The model under review builds one solid part; all positions refer to its coordinate system, in mm. Face numbers are marked on the shaded views. A direction names the side the tool comes from. Give positions to 0.01 mm unless a question says otherwise; leave off trailing zeros. Order: outer loops, then holes, each group sorted by start corner. A loop starts at its lowest first (then second) coordinate and runs counter-clockwise, first axis right, second up.
```python
from build123d import *

# Parameters (mm, degrees)
F1_DEPTH = 82.75
F2_SIZE  = 5
F3_R     = 31
F4_DEPTH = 33
F5_SIZE  = 2
F6_R     = 11.6
F7_DEPTH = 31.5
F8_R     = 32.5
F9_DEPTH = 28
F9_TAPER = 5
F11_D    = 6.6


with BuildPart() as f1:
    # F0 (on Top) → F1 (new body, symmetric)
    with BuildSketch(Plane.XY):
        Polygon((0, 37), (-55, 37), (-55, 25.5), (-40, 25.5), (-40, -36), (0, -36), (40, -36), (40, 25.5), (55, 25.5), (55, 37), align=None)
    extrude(amount=F1_DEPTH, both=True)

    # F2
    f2_edges = [f1.edges().sort_by_distance(p)[0] for p in [
        (40, -36, 0),
        (-40, -36, 0),
    ]]
    chamfer(f2_edges, length=F2_SIZE)

    # F3 (on face) → F4 (join)
    with BuildSketch(Plane(origin=(0, 0, -82.75), x_dir=(1, 0, 0), z_dir=(0, 0, -1))):
        Circle(F3_R)
    extrude(amount=F4_DEPTH)

    # F5
    f5_edges = [f1.edges().sort_by_distance(p)[0] for p in [
        (-31, 0, -115.75),
    ]]
    chamfer(f5_edges, length=F5_SIZE)

    # F6 (on face) → F7 (join)
    with BuildSketch(Plane(origin=(0, 0, -115.75), x_dir=(1, 0, 0), z_dir=(0, 0, -1))):
        Circle(F6_R)
    extrude(amount=F7_DEPTH)

    # F8 (on face) → F9 (join)
    with BuildSketch(Plane.XY.offset(82.75)):
        Circle(F8_R)
    extrude(amount=F9_DEPTH, taper=F9_TAPER)

    # F11 (through all)
    with Locations(Plane.XZ.offset(-25.5)):
        with Locations((-47.5, 52.25), (-47.5, 17.25), (-47.5, -17.75), (-47.5, -52.75), (47.5, 52.25), (47.5, 17.25), (47.5, -17.75), (47.5, -52.75)):
            Hole(F11_D / 2)


solid = f1.part
```
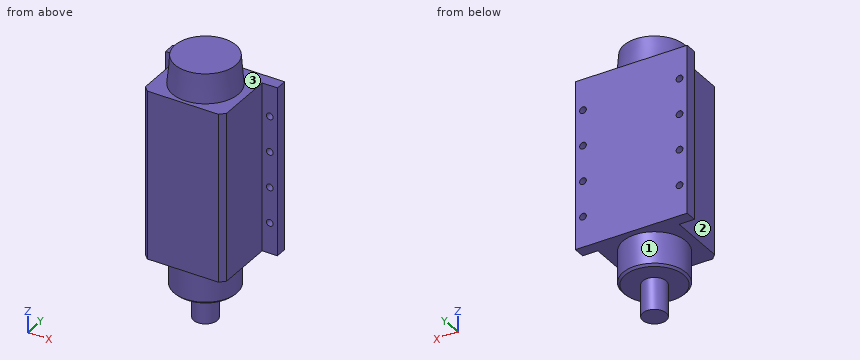
1. Take a section at D-D (z = -39). Write out the cut boundary in (x, y).
2. Take a section at A-A (z = 17.25). Write out the cut boundary in (x, y).
3. For the marked faces 1, 2 and 3, list the 3-axis set-ups (+Z, -Z, +X, -X, +Y, -Y) from which the entire face can be reached by the end or side of a thin tool; tool diameter is ignored.
4. Take a section at B-B (x = -47.5). Write out the cut boundary in (y, z), and give its area (3 significant figures).
5. To check wall thickness, follow line 1 (Z direction, x = -47, y = 30); line 2 (X direction, y = 34, z = 17); line 3 (X direction, y = 31, z = -17). State the ranges of each line that lie inside material, in increasing order.
6. Insertion check: pin 1 (8.5 mm diameter, centred on x = -47.5, z = 52.25, fed in from -Y); pin 2 (4 mm diameter, centred on x = 47.5, z = 52.25, fed in from -Y); pin 3 (5 mm diameter, centred on x = -36, y = -28, fed in from -Z); pin 4 (16.5 mm diameter, centred on x = -47.5, z = 24, fed in from -Y). Each pin has a flat end and moves straight along its axis. Give the tip position at first contact, or say it passes through.
7. Take a section at C-C (y = 0). Write out the cut boundary in (x, z), and give its area (3 significant figures).
Answer:
1. outline: (-55, 25.5) - (-40, 25.5) - (-40, -31) - (-35, -36) - (35, -36) - (40, -31) - (40, 25.5) - (55, 25.5) - (55, 37) - (-55, 37) - close
2. outline: (-55, 25.5) - (-50.8, 25.5) - (-50.8, 37) - (-55, 37) - close; (-44.2, 25.5) - (-40, 25.5) - (-40, -31) - (-35, -36) - (35, -36) - (40, -31) - (40, 25.5) - (44.2, 25.5) - (44.2, 37) - (-44.2, 37) - close; (50.8, 25.5) - (55, 25.5) - (55, 37) - (50.8, 37) - close
3. face 1: -Z
3. face 2: +Z, -Z, -X, -Y
3. face 3: +Z
4. outline: (25.5, -82.75) - (37, -82.75) - (37, -56.05) - (25.5, -56.05) - close; (25.5, -49.45) - (37, -49.45) - (37, -21.05) - (25.5, -21.05) - close; (25.5, -14.45) - (37, -14.45) - (37, 13.95) - (25.5, 13.95) - close; (25.5, 20.55) - (37, 20.55) - (37, 48.95) - (25.5, 48.95) - close; (25.5, 55.55) - (37, 55.55) - (37, 82.75) - (25.5, 82.75) - close
4. area: 1,600 mm2
5. line 1: z = -82.75 to -56.01, -49.49 to -21.01, -14.49 to 13.99, 20.51 to 48.99, 55.51 to 82.75
5. line 2: x = -55 to -50.79, -44.21 to 44.21, 50.79 to 55
5. line 3: x = -55 to -50.71, -44.29 to 44.29, 50.71 to 55
6. pin 1: stops at y = 25.5
6. pin 2: passes through
6. pin 3: stops at z = -82.75
6. pin 4: stops at y = -31.75
7. outline: (-40, -82.75) - (-31, -82.75) - (-31, -113.75) - (-29, -115.75) - (-11.6, -115.75) - (-11.6, -147.25) - (11.6, -147.25) - (11.6, -115.75) - (29, -115.75) - (31, -113.75) - (31, -82.75) - (40, -82.75) - (40, 82.75) - (32.5, 82.75) - (30.05, 110.75) - (-30.05, 110.75) - (-32.5, 82.75) - (-40, 82.75) - close
7. area: 17,800 mm2
